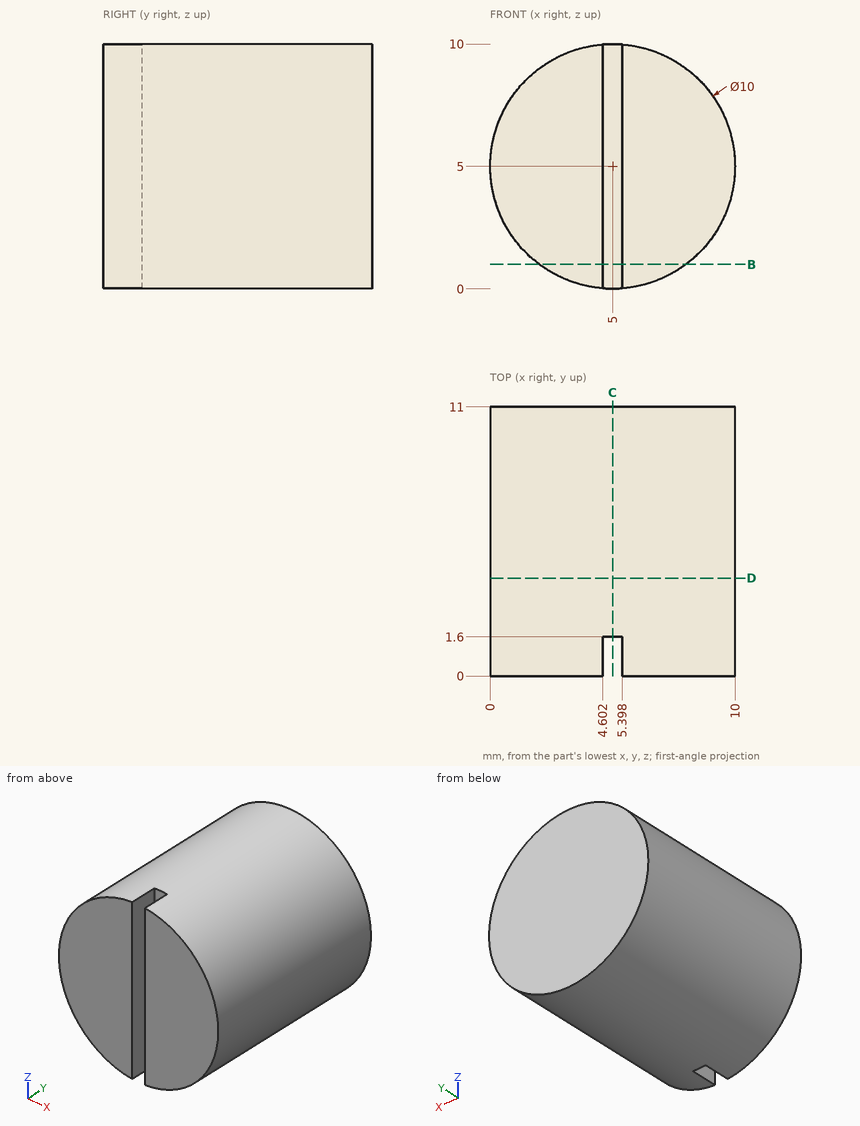
Verification items for this drawing (mm, ordinates from the low corner). Give positions to 0.01 mm unless a question says otherwise; leave off trailing zeros. Loops run counter-clockwise (first coordinate to the right, second up) from the corner with the lowest first, then second, coordinate; pieces in that order, holes last. Notation, with made-up numbers: M 64,32 L 120,32 A25 cw 120,44 Z; hole C -20.75,-15.75 d4. An arc over 180 degrees is marked long. Answer as a JSON object with one key per item and string values. Group by question number.
Item 1: Sectioned sample at D-D on y = 4. Record the boundary of the cut face in (x, z).
Item 2: Sectioned sample at B-B on z = 1. Record the boundary of the cut face in (x, y), plus the area to 3 significant figures.
Item 3: Gauge pin test, flat ends, axial feed: pin 1 (1.3 mm diameter, centred on y = 1, z = 7, fed in from +X); pin 2 (0.5 mm diameter, centred on y = 1, z = 5.5, fed in from -X); pin 3 (3 mm diameter, centred on x = 3, y = 9.5, fed in from +Z). Record the tip position at first contact, or that the pin passes through.
Item 4: Sectioned sample at C-C on x = 5. Record the boundary of the cut face in (y, z), plus the area to 3 significant figures.
Item 5: Material ranges on L1, parallel to Z at x = 0.5, y = 10.75; L2, parallel to Z at x = 6, y = 4; L3, parallel to X at y = 5.5, z = 9, recorded low to high.
Findings below:
{
 "1": {"outline": "C 5,5 d10"},
 "2": {"outline": "M 2,0 L 4.6,0 L 4.6,1.6 L 5.4,1.6 L 5.4,0 L 8,0 L 8,11 L 2,11 Z", "area": "64.7 mm2"},
 "3": {"pin 1": "x = 9.81", "pin 2": "x = 0.01", "pin 3": "z = 9.97"},
 "4": {"outline": "M 1.6,0 L 11,0 L 11,10 L 1.6,10 Z", "area": "94.0 mm2"},
 "5": {"L1": "2.82 to 7.18", "L2": "0.1 to 9.9", "L3": "2 to 8"}
}
